The model under review builds one solid part; all positions refer to its coordinate system, in mm. A direction names the side the tool comes from. Round coordinates to 2 decimals unless told otherwise and drop trailing zeros. Order: outer loops, then holes, each group sorted by start corner. A loop starts at its lowest first (then second) coordinate and runs counter-clockwise, first axis right, second up.
```python
from build123d import *

# Parameters (mm, degrees)
SKETCH1_R               = 40
BOSS_EXTRUDE1_DEPTH     = 106.62
SKETCH2_R               = 44
BOSS_EXTRUDE2_DEPTH     = 16.86
SKETCH3_R               = 38.1
BOSS_EXTRUDE3_DEPTH     = 50
LPATTERN1_COUNT         = 2
LPATTERN1_PITCH         = 66.86
BOSS_EXTRUDE4_START     = -150.688
SKETCH1_2_R             = 40
BOSS_EXTRUDE4_DEPTH     = 66.968
BOSS_EXTRUDE5_DEPTH     = 16.86
SKETCH5_R               = 38.1
BOSS_EXTRUDE6_DEPTH     = 50
LPATTERN2_COUNT         = 2
LPATTERN2_PITCH         = 66.86
BOSS_EXTRUDE7_START     = -304.268
SKETCH1_3_R             = 40
BOSS_EXTRUDE7_DEPTH     = 69.86
BOSS_EXTRUDE8_DEPTH     = 16.86
SKETCH7_R               = 38.1
BOSS_EXTRUDE9_DEPTH     = 50
BOSS_EXTRUDE10_START    = 66.86
BOSS_EXTRUDE10_DEPTH    = 16.86
BOSS_EXTRUDE11_START    = 69.86
SKETCH8_R               = 40
BOSS_EXTRUDE11_DEPTH    = 69.86
SKETCH9_R               = 40
BOSS_EXTRUDE12_DEPTH    = 16.86
SKETCH10_R              = 38.1
BOSS_EXTRUDE13_DEPTH    = 50
BOSS_EXTRUDE14_START    = 66.86
SKETCH9_3_R             = 40
BOSS_EXTRUDE14_DEPTH    = 16.86
BOSS_EXTRUDE15_START    = 193.44
SKETCH9_4_R             = 40
BOSS_EXTRUDE15_DEPTH    = 109.72
CUT_EXTRUDE1_DEPTH      = 669.804560177
CUT_EXTRUDE1_DEPTH_BACK = 669.804560177
CUT_EXTRUDE2_DEPTH      = 669.804560177
CUT_EXTRUDE2_DEPTH_BACK = 669.804560177


with BuildPart() as part:
    # Sketch1 → Boss-Extrude1 (new body)
    with BuildSketch(Plane(origin=(0, 0, 0), x_dir=(0, 0, -1), z_dir=(1, 0, 0))):
        Circle(SKETCH1_R)
    extrude(amount=BOSS_EXTRUDE1_DEPTH)

    # Sketch2 → Boss-Extrude2 (add)
    with BuildSketch(Plane(origin=(0, 0, 0), x_dir=(0, 0, -1), z_dir=(1, 0, 0))):
        with BuildLine():
            Line((52.203036807, 7.220314961), (43.585078169, 69.528346457))
            ThreePointArc((43.585078169, 69.528346457), (43.89614698, 66.521304401), (44, 63.5))
            ThreePointArc((44, 63.5), (-3.021304401, 19.60385302), (-43.585078169, 69.528346457))
            Line((-43.585078169, 69.528346457), (-52.203036807, 7.220314961))
            ThreePointArc((-52.203036807, 7.220314961), (-52.575612406, 3.61869868), (-52.7, 0))
            Line((-52.7, 0), (-90.932667397, -52.5))
            ThreePointArc((-90.932667397, -52.5), (0, -105), (90.932667397, -52.5))
            Line((90.932667397, -52.5), (52.7, 0))
            ThreePointArc((52.7, 0), (52.575612406, 3.61869868), (52.203036807, 7.220314961))
        make_face()
        with Locations((0, 63.5)):
            Circle(SKETCH2_R)
    boss_extrude2 = extrude(amount=-BOSS_EXTRUDE2_DEPTH)

    # Sketch3 → Boss-Extrude3 (add)
    with BuildSketch(Plane.ZY.offset(16.86)):
        with Locations(Location((0, 63.5, 0), (0, 0, 180))):
            Circle(SKETCH3_R)
    extrude(amount=BOSS_EXTRUDE3_DEPTH)

    # LPattern1: Boss-Extrude2 ×2
    with Locations(*[(-i * LPATTERN1_PITCH, 0, 0) for i in range(1, LPATTERN1_COUNT)]):
        add(boss_extrude2)

    # Sketch1<2> → Boss-Extrude4 (add)
    with BuildSketch(Plane(origin=(0, 0, 0), x_dir=(0, 0, -1), z_dir=(1, 0, 0)).offset(BOSS_EXTRUDE4_START)):
        Circle(SKETCH1_2_R)
    extrude(amount=BOSS_EXTRUDE4_DEPTH)

    # Sketch4 → Boss-Extrude5 (add)
    with BuildSketch(Plane.ZY.offset(150.688)):
        with BuildLine():
            Line((-7.602260115, 52.148783698), (-63.5, 44))
            ThreePointArc((-63.5, 44), (-107.5, 0), (-63.5, -44))
            Line((-63.5, -44), (-7.602260115, -52.148783698))
            ThreePointArc((-7.602260115, -52.148783698), (52.7, 0), (-7.602260115, 52.148783698))
        make_face()
    boss_extrude5 = extrude(amount=BOSS_EXTRUDE5_DEPTH)

    # Sketch5 → Boss-Extrude6 (add)
    with BuildSketch(Plane.ZY.offset(167.548)):
        with Locations((-63.5, 0)):
            Circle(SKETCH5_R)
    extrude(amount=BOSS_EXTRUDE6_DEPTH)

    # LPattern2: Boss-Extrude5 ×2
    with Locations(*[(-i * LPATTERN2_PITCH, 0, 0) for i in range(1, LPATTERN2_COUNT)]):
        add(boss_extrude5)

    # Sketch1<3> → Boss-Extrude7 (add)
    with BuildSketch(Plane(origin=(0, 0, 0), x_dir=(0, 0, -1), z_dir=(1, 0, 0)).offset(BOSS_EXTRUDE7_START)):
        Circle(SKETCH1_3_R)
    extrude(amount=BOSS_EXTRUDE7_DEPTH)

    # Sketch6 → Boss-Extrude8 (add)
    with BuildSketch(Plane.ZY.offset(304.268)):
        with BuildLine():
            Line((7.653321337, -52.148783698), (63.551061222, -44))
            ThreePointArc((63.551061222, -44), (107.551061222, 0), (63.551061222, 44))
            Line((63.551061222, 44), (7.653321337, 52.148783698))
            ThreePointArc((7.653321337, 52.148783698), (-52.648938778, 0), (7.653321337, -52.148783698))
        make_face()
    extrude(amount=BOSS_EXTRUDE8_DEPTH)

    # Sketch7 → Boss-Extrude9 (add)
    with BuildSketch(Plane.ZY.offset(321.128)):
        with Locations((63.551061222, 0)):
            Circle(SKETCH7_R)
    extrude(amount=BOSS_EXTRUDE9_DEPTH)

    # Sketch6<2> → Boss-Extrude10 (add)
    with BuildSketch(Plane.ZY.offset(304.268).offset(BOSS_EXTRUDE10_START)):
        with BuildLine():
            Line((7.653321337, -52.148783698), (63.551061222, -44))
            ThreePointArc((63.551061222, -44), (107.551061222, 0), (63.551061222, 44))
            Line((63.551061222, 44), (7.653321337, 52.148783698))
            ThreePointArc((7.653321337, 52.148783698), (-52.648938778, 0), (7.653321337, -52.148783698))
        make_face()
    extrude(amount=BOSS_EXTRUDE10_DEPTH)

    # Sketch8 → Boss-Extrude11 (add)
    with BuildSketch(Plane.ZY.offset(387.988).offset(BOSS_EXTRUDE11_START)):
        with Locations(Location((0, 0, 0), (0, 0, 180))):
            Circle(SKETCH8_R)
    extrude(amount=-BOSS_EXTRUDE11_DEPTH)

    # Sketch9 → Boss-Extrude12 (add)
    # profile 1 of 2: a face of its own
    with BuildSketch(Plane.ZY.offset(457.848)):
        with BuildLine():
            Line((52.7, 0), (90.932667397, 52.5))
            ThreePointArc((90.932667397, 52.5), (0, 105), (-90.932667397, 52.5))
            Line((-90.932667397, 52.5), (-52.7, 0))
            ThreePointArc((-52.7, 0), (-52.575612406, -3.61869868), (-52.203036807, -7.220314961))
            Line((-52.203036807, -7.220314961), (-43.585078169, -69.528346457))
            ThreePointArc((-43.585078169, -69.528346457), (0, -107.5), (43.585078169, -69.528346457))
            Line((43.585078169, -69.528346457), (52.203036807, -7.220314961))
            ThreePointArc((52.203036807, -7.220314961), (52.575612406, -3.61869868), (52.7, 0))
        make_face()
        with Locations(Location((0, 0, 0), (0, 0, 180))):
            Circle(SKETCH9_R, mode=Mode.SUBTRACT)
    # profile 2 of 2: a face of its own
    with BuildSketch(Plane.ZY.offset(457.848)):
        with Locations(Location((0, 0, 0), (0, 0, 180))):
            Circle(SKETCH9_R)
    extrude(amount=BOSS_EXTRUDE12_DEPTH)

    # Sketch10 → Boss-Extrude13 (add)
    with BuildSketch(Plane.ZY.offset(474.708)):
        with Locations((0, -63.5)):
            Circle(SKETCH10_R)
    extrude(amount=BOSS_EXTRUDE13_DEPTH)

    # Sketch9<3> → Boss-Extrude14 (add)
    # profile 1 of 2: a face of its own
    with BuildSketch(Plane.ZY.offset(457.848).offset(BOSS_EXTRUDE14_START)):
        with BuildLine():
            Line((52.7, 0), (90.932667397, 52.5))
            ThreePointArc((90.932667397, 52.5), (0, 105), (-90.932667397, 52.5))
            Line((-90.932667397, 52.5), (-52.7, 0))
            ThreePointArc((-52.7, 0), (-52.575612406, -3.61869868), (-52.203036807, -7.220314961))
            Line((-52.203036807, -7.220314961), (-43.585078169, -69.528346457))
            ThreePointArc((-43.585078169, -69.528346457), (0, -107.5), (43.585078169, -69.528346457))
            Line((43.585078169, -69.528346457), (52.203036807, -7.220314961))
            ThreePointArc((52.203036807, -7.220314961), (52.575612406, -3.61869868), (52.7, 0))
        make_face()
        with Locations(Location((0, 0, 0), (0, 0, 180))):
            Circle(SKETCH9_3_R, mode=Mode.SUBTRACT)
    # profile 2 of 2: a face of its own
    with BuildSketch(Plane.ZY.offset(457.848).offset(BOSS_EXTRUDE14_START)):
        with Locations(Location((0, 0, 0), (0, 0, 180))):
            Circle(SKETCH9_3_R)
    extrude(amount=BOSS_EXTRUDE14_DEPTH)

    # Sketch9<4> → Boss-Extrude15 (add)
    with BuildSketch(Plane.ZY.offset(457.848).offset(BOSS_EXTRUDE15_START)):
        with Locations(Location((0, 0, 0), (0, 0, 180))):
            Circle(SKETCH9_4_R)
    extrude(amount=-BOSS_EXTRUDE15_DEPTH)

    # Sketch11 → Cut-Extrude1 (cut, two sides: drawn at the far end of the back side and taken through both)
    with BuildSketch(Plane.XY.offset(-CUT_EXTRUDE1_DEPTH_BACK)):
        Polygon((-533.138, 105), (-524.708, 105), (-524.708, 26.25), align=None)
        Polygon((-474.708, 105), (-466.278, 105), (-474.708, 26.25), align=None)
        Polygon((-541.568, -107.5), (-533.138, -107.5), (-541.568, -58.5), align=None)
        Polygon((-466.278, -107.5), (-457.848, -107.5), (-457.848, -58.5), align=None)
        Polygon((-75.29, -105), (-66.86, -26.25), (-66.86, -105), align=None)
        Polygon((-16.86, -26.25), (-8.43, -105), (-16.86, -105), align=None)
        Polygon((-8.43, 107.5), (0, 107.5), (0, 58.5), align=None)
        Polygon((-83.72, 107.5), (-75.29, 107.5), (-83.72, 58.5), align=None)
    extrude(amount=CUT_EXTRUDE1_DEPTH + CUT_EXTRUDE1_DEPTH_BACK, mode=Mode.SUBTRACT)

    # Sketch12 → Cut-Extrude2 (cut, two sides: drawn at the far end of the back side and taken through both)
    with BuildSketch(Plane(origin=(0, 0, 0), x_dir=(1, 0, 0), z_dir=(0, 1, 0)).offset(-CUT_EXTRUDE2_DEPTH_BACK)):
        Polygon((-379.558, -107.551061222), (-387.988, -58.551061222), (-387.988, -107.551061222), align=None)
        Polygon((-304.268, -107.551061222), (-304.268, -58.551061222), (-312.698, -107.551061222), align=None)
        Polygon((-379.558, 52.648938778), (-371.128, 52.648938778), (-371.128, 22.49780872), align=None)
        Polygon((-312.698, 52.648938778), (-321.128, 22.49780872), (-321.128, 52.648938778), align=None)
        Polygon((-159.118, 107.5), (-150.688, 107.5), (-150.688, 58.5), align=None)
        Polygon((-225.978, 107.5), (-234.408, 107.5), (-234.408, 58.5), align=None)
        Polygon((-217.548, -52.7), (-225.978, -52.7), (-217.548, -22.548869942), align=None)
        Polygon((-159.118, -52.7), (-167.548, -22.548869942), (-167.548, -52.7), align=None)
    extrude(amount=CUT_EXTRUDE2_DEPTH + CUT_EXTRUDE2_DEPTH_BACK, mode=Mode.SUBTRACT)


solid = part.part
```
(1) Consider section D-D (y = -78). Write out the cut boundary in (x, z).
Data:
outline: (-538.21, -41.54) - (-524.71, -41.54) - (-524.71, -35.23) - (-474.71, -35.23) - (-474.71, -41.54) - (-461.2, -41.54) - (-461.2, 41.54) - (-474.71, 41.54) - (-474.71, 35.23) - (-524.71, 35.23) - (-524.71, 41.54) - (-538.21, 41.54) - close; (-83.72, -70.29) - (-72.4, -70.29) - (-72.4, 70.29) - (-83.72, 70.29) - close; (-11.32, -70.29) - (0, -70.29) - (0, 70.29) - (-11.32, 70.29) - close
(2) Draft analysis for pull direction X (two halves, no side actions). For faces 1 (the flat face through (106.62, 1, 1)), 2 (the flat face through (-466.16, 25.883, 71.549)), 3 (the flat face through (-379.44, -48.13, 35.21)), state which applies: pulls with the +X half, pulls with the -X half, needs draft (parallel to the pull), parting line crosses it, or undercut.
Data:
face 1: pulls with the +X half
face 2: needs draft
face 3: undercut
(3) To check wall thickness, follow probe 1 along X at (y, z) = (-19, -11); probe 2 along X at (y, z) = (53, -45.5); probe 3 along X at (y, z) = (-4, -32). State the ranges of each line that lie inside material, in increasing order.
Data:
probe 1: x = -651.29 to -524.71, -474.71 to -371.13, -321.13 to -217.55, -167.55 to -66.86, -16.86 to 106.62
probe 2: x = -541.57 to -527.57, -471.84 to -457.85, -83.72 to -66.86, -16.86 to 0
probe 3: x = -651.29 to -524.71, -474.71 to -373.78, -318.47 to -66.86, -16.86 to 106.62
(4) Consider section C-C (z = 0). State how many separate pieces and enclosed holes the cut face has, and give its area (3 significant figures).
Data:
separate pieces: 3
enclosed holes: 0
area: 60,700 mm2
(5) Insertion check: pin 1 (3 mm diameter, centred on x = -475.5, z = 29.5, fed in from -Y); pin 2 (3 mm diameter, centred on x = -523.5, z = 9.5, fed in from -Y); pin 3 (2 mm diameter, centred on x = -225, z = 36.5, fed in from +Y). Each pin has a flat end and moves straight along its axis. Give the tip position at first contact, or say it passes through.
Data:
pin 1: stops at y = -97.25
pin 2: stops at y = -106.65
pin 3: stops at y = 38.95
(6) Consider section B-B (x = -593). Write out the cut boundary in (y, z).
Data:
outline: circle Ø80 at (0, 0)
(7) Consider section A-A (y = 79). Write out the cut boundary in (x, z), and give its area (3 significant figures).
Data:
outline: (-541.57, -69.17) - (-530.35, -69.17) - (-530.35, 69.17) - (-541.57, 69.17) - close; (-469.06, -69.17) - (-457.85, -69.17) - (-457.85, 69.17) - (-469.06, 69.17) - close; (-80.19, -41.18) - (-66.86, -41.18) - (-66.86, -34.8) - (-16.86, -34.8) - (-16.86, -41.18) - (-3.53, -41.18) - (-3.53, 41.18) - (-16.86, 41.18) - (-16.86, 34.8) - (-66.86, 34.8) - (-66.86, 41.18) - (-80.19, 41.18) - close
area: 8,780 mm2
(8) For faces 4 (the flat face through (-159, 48.13, -35.16)), 5 (the flat face through (-217.548, 1, -14)), 6 (the cylindrical face through (52.56, -39.05, 8.67)), 7 (the flat face through (-164.21, -0.67, 34.49)), 8 (the cylindrical face through (-72.57, 107.49, -0.88)), list the 3-axis set-ups (+Z, -Z, +X, -X, +Y, -Y) from which the entire face can be reached by the end or side of a thin tool; tool diameter is ignored.
Data:
face 4: -Z, +Y
face 5: none
face 6: +X
face 7: +Z, +Y, -Y
face 8: +X, +Y
